from build123d import *

# Parameters (mm, degrees)
F0_W     = 70
F0_H     = 70
F1_DEPTH = 500
F2_W     = 18
F2_H     = 40
F3_DEPTH = 40
F4_SIZE  = 5


with BuildPart() as f1:
    # F0 (on Right) → F1 (new body)
    with BuildSketch(Plane.YZ):
        Rectangle(F0_W, F0_H)
    extrude(amount=F1_DEPTH)

    # F2 (on face) → F3 (join)
    with BuildSketch(Plane(origin=(0, 0, 0), x_dir=(0, -1, 0), z_dir=(-1, 0, 0))):
        Rectangle(F2_W, F2_H)
    extrude(amount=F3_DEPTH)

    # F4
    f4_edges = [f1.edges().sort_by_distance(p)[0] for p in [
        (250, -35, 35),
        (250, 35, 35),
        (250, -35, -35),
    ]]
    chamfer(f4_edges, length=F4_SIZE)


solid = f1.part
The listing builds one solid part. Answer for the finished solid, in the listing's coordinates (mm). A direction names the side the tool comes from. Coordinates: 2 decimals unless noted, no trailing zeros. Loops run counter-clockwise (first coordinate to the right, second up) from the corner with the lowest first, then second, coordinate; pieces in that order, holes last. Notation, with made-up numbers: (45, -5.75) -> (69, -5.75) arc R26 cw to (69, 30.25) -> close; hole circle Ø4 at (77, 87.5). An arc over 180 degrees is marked (long way). Answer in a Markdown table with one row per item. Add a question column.
1. The part is cut by section B-B, the plane y = 3.5. Write down the section's boundary in (x, z), then the cut area to 3 significant figures.
2. For faces 1 (the flat face through (-20, 9, 0)), 2 (the flat face through (-20, 0, 20)), 3 (the flat face through (-20, -9, 0)), 4 (the flat face through (-20, 0, -20)), 5 (the flat face through (246, 0, 35)), determine the directions among +Z, -Z, +X, -X, +Y, -Y from which every point of the face is accessible in a straight line to the end or side of a thin tool.
3. The part is cut by section C-C, the plane z = 24.5. Write down the section's boundary in (x, y), then the cut area to 3 significant figures.
4. The part is cut by section A-A, the plane z = 2. Write down the section's boundary in (x, y).
5. Consider line 1 (X direction, y = -22, z = 15.5). Determine where the line is inside the solid, lowest interval first. Write a range as [from, to].
6. Flat-ended cylindrical pins translate along their axes: P1, Ø8, axis at y = 24, z = -6, coming from the -X side; P2, Ø14.5, axis at x = -27, y = 4, coming from the +Z side; P3, Ø14.5, axis at x = -28, y = -1.5, coming from the -Z side. Find the tip coordinate at first contact, or state that the pin passes through.
Answer below:
| question | item | result |
|---|---|---|
| 1 | outline | (-40, -20) -> (0, -20) -> (0, -35) -> (500, -35) -> (500, 35) -> (0, 35) -> (0, 20) -> (-40, 20) -> close |
| 1 | area | 36,600 mm2 |
| 2 | face 1 | +Z, -Z, -X, +Y |
| 2 | face 2 | +Z, -X, +Y, -Y |
| 2 | face 3 | +Z, -Z, -X, -Y |
| 2 | face 4 | -Z, -X, +Y, -Y |
| 2 | face 5 | +Z, +X, -X, +Y, -Y |
| 3 | outline | (0, -35) -> (500, -35) -> (500, 35) -> (0, 35) -> close |
| 3 | area | 35,000 mm2 |
| 4 | outline | (-40, -9) -> (0, -9) -> (0, -35) -> (500, -35) -> (500, 35) -> (0, 35) -> (0, 9) -> (-40, 9) -> close |
| 5 | line 1 | [0, 500] |
| 6 | P1 | x = 0 |
| 6 | P2 | z = 20 |
| 6 | P3 | z = -20 |
